The listing builds one solid part. Answer for the finished solid, in the listing's coordinates (mm). Face numbers are marked on the shaded views. A direction names the side the tool comes from. Round coordinates to 2 decimals unless told otherwise and drop trailing zeros. Order: outer loops, then holes, each group sorted by start corner. A loop starts at its lowest first (then second) coordinate and runs counter-clockwise, first axis right, second up. Notation, with made-up numbers: (59, 72) - (87, 72) arc R25 cw to (87, 96) - close; hole circle Ø4 at (-23, 1). An arc over 180 degrees is marked (long way). Use CSV: the item, a comma, the result in double quotes. Start each with the question number.
Item 1: Find section D-D, the plane z = 3.75. Give the vertices of the cut face in (x, y).
Item 2: Straight lines are drawn through the part: line 1 along Y through (x, z) = (2, 7.5); line 2 along Y through (x, z) = (10.5, 2.5); line 3 along Z through (x, y) = (32, -71). For each, find the intervals that lie inside material, in ascending order. Write a range as [from, to].
Item 3: Flat-ended cylindrical pins translate along their axes: P1, Ø7.5, axis at y = -37.5, z = 4.5, coming from the +X side; P2, Ø8, axis at x = 29.5, y = -63.5, coming from the +Z side. Find the tip coordinate at first contact, or state that the pin passes through.
Item 4: Find section C-C, the plane x = 31.5. Give the vertices of the cut face in (y, z).
Item 5: Find section B-B, the plane y = -44. Give the vertices of the cut face in (x, z), plus the area to 3 significant figures.
Item 6: Determine the mould class of the marked faces 1, 2 and 3 for opening direction X: +X half, -X half, draft (parallel to the pull), parting line (faces both ways), or undercut.
Item 7: Find section A-A, the plane x = 11. Give the vertices of the cut face in (y, z), plus the area to 3 significant figures.
Item 8: For the marked faces 4 and 5, determine the directions among +Z, -Z, +X, -X, +Y, -Y from which every point of the face is accessible in a straight line to the end or side of a thin tool.
Autodesk Inventor part; units mm, degrees
ref_plane "YZ Plane" through (0, 0, 0) normal (1, 0, 0) x (0, 1, 0)
ref_plane "XZ Plane" through (0, 0, 0) normal (0, 1, 0) x (-1, 0, 0)
ref_plane "XY Plane" through (0, 0, 0) normal (0, 0, 1) x (1, 0, 0)
sketch "Sketch1" plane through (0, 0, 0) normal (0, 0, 1) x (1, 0, 0)
  line L0 (0, 0) -> (0, -82)
  line L1 (0, -82) -> (15, -82)
  line L2 (15, -82) -> (15, -75) construction
  line L3 (15, -75) -> (38, -75) construction
  line L4 (15, -82) -> (38, -75)
  line L5 (38, -75) -> (38, -69)
  line L6 (38, -69) -> (10, -69)
  line L7 (10, -69) -> (10, -17)
  line L8 (10, -17) -> (38, -17)
  line L9 (38, -17) -> (38, -11)
  line L10 (0, 0) -> (15, 0)
  line L11 (15, 0) -> (38, -11)
  dimension "d0" = 82
  dimension "d1" = 15
  dimension "d2" = 90
  dimension "d3" = 7
  dimension "d4" = 23
  dimension "d5" = 6
  dimension "d6" = 28
  dimension "d7" = 90
  dimension "d8" = 52
  dimension "d9" = 90
  dimension "d10" = 28
  dimension "d11" = 6
  dimension "d12" = 15
extrude "Extrusion1" add sketch "Sketch1" along normal blind 15
sketch "Sketch2" plane through (10, -69, 0) normal (0, 1, 0) x (1, 0, 0)
  line L0 (5, 0) -> (28, 0)
  line L1 (28, 0) -> (28, -15)
  line L2 (5, -15) -> (28, -15)
  line L3 (5, 0) -> (5, -15)
  line L4 (28, 0) -> (28, -15) construction
  line L5 (28, -7.5) -> (22, -7.5) construction
  circle A0 centre (22, -7.5) radius 3
  point P0 (-10, 0)
  dimension "d15" = 6
  dimension "d16" = 6
extrude "Extrusion2" cut sketch "Sketch2" against normal blind 15 contours A0
sketch "Sketch3" plane through (10, -69, 0) normal (1, 0, 0) x (0, 0, -1)
  line L0 (0, 52) -> (-15, 52) construction
  line L1 (-7.5, 52) -> (-7.5, 35) construction
  line L2 (-7.5, 52) -> (9.5, 52) construction
  line L3 (-7.5, 35) -> (-7.5, 25) construction
  circle A0 centre (-7.5, 35) radius 2.5
  circle A1 centre (-7.5, 25) radius 2.5
  point P0 (0, 69)
  dimension "d19" = 17
  dimension "d20" = 90
  dimension "d21" = 10
  dimension "d22" = 5
  dimension "d23" = 5
extrude "Extrusion3" cut sketch "Sketch3" against normal blind 15
properties part number "clamp"
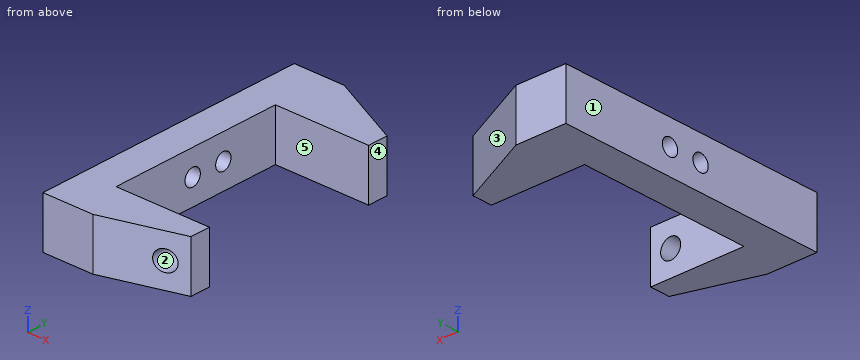
Worked out:
1,outline,"(0, -82) - (15, -82) - (38, -75) - (38, -69) - (10, -69) - (10, -17) - (38, -17) - (38, -11) - (15, 0) - (0, 0) - close"
2,line 1,"y = [-82, -46.5], [-41.5, -36.5], [-31.5, 0]"
2,line 2,"y = [-82, -69], [-17, 0]"
2,line 3,"z = [0, 4.5], [10.5, 15]"
3,P1,"stops at x = 10"
3,P2,"passes through"
4,outline,"(-76.98, 0) - (-69, 0) - (-69, 4.54) - (-76.98, 4.54) - close; (-76.98, 10.46) - (-69, 10.46) - (-69, 15) - (-76.98, 15) - close; (-17, 0) - (-7.89, 0) - (-7.89, 15) - (-17, 15) - close"
5,outline,"(0, 0) - (10, 0) - (10, 5) - (0, 5) - close; (0, 10) - (10, 10) - (10, 15) - (0, 15) - close"
5,area,"100 mm²"
6,face 1,"-X half"
6,face 2,"undercut"
6,face 3,"+X half"
7,outline,"(-82, 0) - (-69, 0) - (-69, 15) - (-82, 15) - close; (-17, 0) - (0, 0) - (0, 15) - (-17, 15) - close"
7,area,"450 mm²"
8,face 4,"+Z, -Z, +X, +Y, -Y"
8,face 5,"+Z, -Z, +X"
